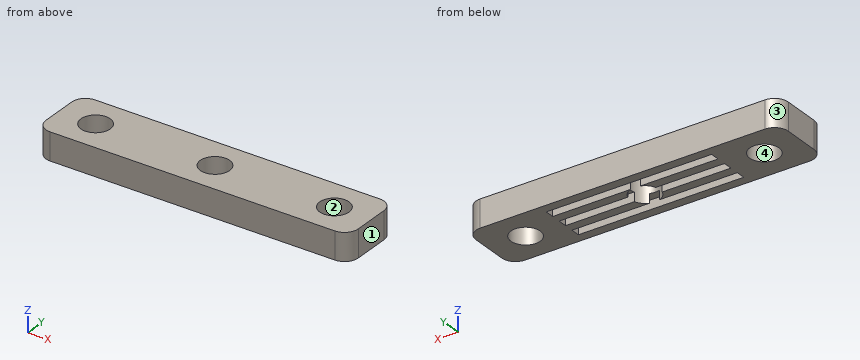
from build123d import *

# Parameters (mm, degrees)
SKETCH1_W           = 34
SKETCH1_H           = 7
SKETCH1_R           = 1.6
BOSS_EXTRUDE1_DEPTH = 3
SKETCH2_W           = 18
SKETCH2_H           = 1
CUT_EXTRUDE1_DEPTH  = 1
FILLET1_R           = 1.5


with BuildPart() as part:
    # Sketch1 → Boss-Extrude1 (new body)
    with BuildSketch(Plane.XY):
        with Locations((17, 3.5)):
            Rectangle(SKETCH1_W, SKETCH1_H)
        with Locations((4, 3.5)):
            Circle(SKETCH1_R, mode=Mode.SUBTRACT)
        with Locations((30, 3.5)):
            Circle(SKETCH1_R, mode=Mode.SUBTRACT)
        with Locations((17, 3.5)):
            Circle(SKETCH1_R, mode=Mode.SUBTRACT)
    extrude(amount=BOSS_EXTRUDE1_DEPTH)

    # Sketch2 → Cut-Extrude1 (cut)
    with BuildSketch(Plane(origin=(0, 0, 0), x_dir=(-1, 0, 0), z_dir=(0, 0, -1))):
        with Locations((-17, 7.5)):
            Rectangle(SKETCH2_W, SKETCH2_H)
        with Locations((-17, 5.5)):
            Rectangle(SKETCH2_W, SKETCH2_H)
        with Locations((-17, 3.5)):
            Rectangle(SKETCH2_W, SKETCH2_H)
        with Locations((-17, 1.5)):
            Rectangle(SKETCH2_W, SKETCH2_H)
        with Locations((-17, -0.5)):
            Rectangle(SKETCH2_W, SKETCH2_H)
    extrude(amount=-CUT_EXTRUDE1_DEPTH, mode=Mode.SUBTRACT)

    # Fillet1
    fillet1_edges = [part.edges().sort_by_distance(p)[0] for p in [
        (0, 7, 1.5),
        (34, 7, 1.5),
        (34, 0, 1.5),
        (0, 0, 1.5),
    ]]
    fillet(fillet1_edges, radius=FILLET1_R)


solid = part.part
Could you check a few things on this model? Use its own coordinates, in mm. Face numbers are marked on the shaded views. Round coordinates to 2 decimals unless told otherwise and drop trailing zeros. Write each loop counter-clockwise with the first axis right and the second up, starting at its lowest first coordinate (ties: lowest second). Pieces come first, ordered by that corner, then holes. Notation, with made-up numbers: (22, 34) -> (48, 34) arc R26 cw to (48, 61) -> close; hole circle Ø6 at (82, -13). An arc over 180 degrees is marked (long way). Use a Markdown table: item, result.
1. If we section it at A-A (x = 17): List the corners of the cut face in (y, z) for me.
Answer key:
| item | result |
|---|---|
| outline | (0, 0) -> (1, 0) -> (1, 1) -> (1.9, 1) -> (1.9, 3) -> (0, 3) -> close; (5.1, 1) -> (6, 1) -> (6, 0) -> (7, 0) -> (7, 3) -> (5.1, 3) -> close |
2. If we section it at C-C (z = 1.4): List the corners of the cut face in (x, y) for me.
Answer key:
| item | result |
|---|---|
| outline | (0, 1.5) arc R1.5 ccw to (1.5, 0) -> (32.5, 0) arc R1.5 ccw to (34, 1.5) -> (34, 5.5) arc R1.5 ccw to (32.5, 7) -> (1.5, 7) arc R1.5 ccw to (0, 5.5) -> close; hole circle Ø3.2 at (4, 3.5); hole circle Ø3.2 at (17, 3.5); hole circle Ø3.2 at (30, 3.5) |
3. If we section it at D-D (x = 25): List the corners of the cut face in (y, z) for me.
Answer key:
| item | result |
|---|---|
| outline | (0, 0) -> (1, 0) -> (1, 1) -> (2, 1) -> (2, 0) -> (3, 0) -> (3, 1) -> (4, 1) -> (4, 0) -> (5, 0) -> (5, 1) -> (6, 1) -> (6, 0) -> (7, 0) -> (7, 3) -> (0, 3) -> close |
4. We'd pull the mould along Y, two halves only. Please class the marked faces 1, 2, 3 and 4: +Y half, -Y half, draft (parallel to the pull), parting line (faces both ways), or undercut.
Answer key:
| item | result |
|---|---|
| face 1 | draft |
| face 2 | undercut |
| face 3 | +Y half |
| face 4 | undercut |
5. For pin 1 Ø1 at (y, z) = (6.5, 2) entering from -X; pin 2 Ø0.8 at (x, y) = (14.5, 5.5) entering from -Z, each with a flat end and sliding along its axis, tell me the tip position at first contact or that it passes through.
Answer key:
| item | result |
|---|---|
| pin 1 | stops at x = 0.09 |
| pin 2 | stops at z = 1 |
6. If we section it at B-B (y = 3.5): List the corners of the cut face in (x, z) for me.
Answer key:
| item | result |
|---|---|
| outline | (0, 0) -> (2.4, 0) -> (2.4, 3) -> (0, 3) -> close; (5.6, 0) -> (8, 0) -> (8, 1) -> (15.4, 1) -> (15.4, 3) -> (5.6, 3) -> close; (18.6, 1) -> (26, 1) -> (26, 0) -> (28.4, 0) -> (28.4, 3) -> (18.6, 3) -> close; (31.6, 0) -> (34, 0) -> (34, 3) -> (31.6, 3) -> close |
7. Please list where these lines run through material, in increasing order: probe 1 along Y at (x, z) = (30, 1.1); probe 2 along X at (y, z) = (4.25, 1.9); probe 3 along Y at (x, z) = (17, 0.85).
Answer key:
| item | result |
|---|---|
| probe 1 | y = 0 to 1.9, 5.1 to 7 |
| probe 2 | x = 0 to 2.59, 5.41 to 15.59, 18.41 to 28.59, 31.41 to 34 |
| probe 3 | y = 0 to 1, 6 to 7 |
